Autodesk Fusion 360 part; units mm, degrees
sketch "Sketch1" plane through (0, 0, 0) normal (0, 0, 1) x (1, 0, 0)
  line L0 (0, 0) -> (36, 0)
  line L1 (36, 0) -> (36, 18)
  line L2 (36, 18) -> (0, 18)
  line L3 (0, 18) -> (0, 0)
  dimension "d1" = 36
  dimension "d2" = 18
extrude "Extrude1" add sketch "Sketch1" along normal blind 20
sketch "Sketch2" plane through (0, 0, 20) normal (0, 0, 1) x (-1, 0, 0)
  line L0 (0, -18) -> (0, 0)
  line L1 (0, 0) -> (-36, 0)
  line L2 (-36, 0) -> (-36, -18)
  line L3 (-36, -18) -> (0, -18)
  circle A0 centre (-18, -18) radius 13
  dimension "d5" = 26
extrude "Extrude2" cut sketch "Sketch2" against normal blind 20 contours L3 A0 picked at (-19.0768, -11.2377)
ref_plane "WorkPlane1" through (0, 20, 0) normal (0, 1, 0) x (0, 0, 1)
sketch "Sketch3" plane through (36, 0, 0) normal (1, 0, 0) x (0, 1, 0)
  line L0 (0, 0) -> (18, 0)
  line L1 (18, 0) -> (18, 20)
  line L2 (18, 20) -> (0, 20)
  line L3 (0, 20) -> (0, 0)
  line L4 (18, 20) -> (15, 20)
  line L5 (15, 20) -> (15, 0)
  line L6 (15, 0) -> (18, 0)
  line L7 (18, 0) -> (18, 20)
extrude "Extrude3" add sketch "Sketch3" along normal blind 5 contours L0 L1 L2 L4 L5 L6 L7
sketch "Sketch4" plane through (0, 0, 0) normal (-1, 0, 0) x (0, -1, 0)
  line L0 (-18, 0) -> (0, 0)
  line L1 (0, 0) -> (0, 20)
  line L2 (0, 20) -> (-18, 20)
  line L3 (-18, 20) -> (-18, 0)
  line L4 (-18, 20) -> (-15, 20)
  line L5 (-15, 20) -> (-15, 0)
  line L6 (-15, 0) -> (-18, 0)
  line L7 (-18, 0) -> (-18, 20)
  point P0 (-15, 0)
extrude "Extrude4" add sketch "Sketch4" along normal blind 5 contours L0 L2 L3 L4 L5 L6 L7
sketch "Sketch5" plane through (0, 15, 0) normal (0, -1, 0) x (1, 0, 0)
  line L0 (36, 20) -> (36, 0)
  line L1 (36, 0) -> (41, 0)
  line L2 (41, 0) -> (41, 20)
  line L3 (41, 20) -> (36, 20)
  line L4 (36, 10) -> (46, 10) construction
  circle A0 centre (38.5, 15) radius 1.5
  line L5 (5, 20) -> (5, 0)
  line L6 (18, 10) -> (18, 25) construction
  circle A1 centre (38.5, 5) radius 1.5
  circle A2 centre (-2.5, 15) radius 1.5
  circle A3 centre (-2.5, 5) radius 1.5
  point P0 (0, 20)
  dimension "d13" = 3
  dimension "d14" = 5
  dimension "d15" = 2.5
Check sheet for the modelled part. Datum: model origin and axes. Units: mm. A direction names the side the tool comes from. Round coordinates to 2 decimals unless told otherwise and drop trailing zeros. Write each loop counter-clockwise with the first axis right and the second up, starting at its lowest first coordinate (ties: lowest second). Pieces come first, ordered by that corner, then holes. Notation, with made-up numbers: (69.25, 53) -> (96.25, 53) arc R20 cw to (96.25, 89) -> close; hole circle Ø4 at (-7.5, 44). An arc over 180 degrees is marked (long way). One line per question, with ' | ' between items. Start each with the question number.
1. Set-up check for faces 1 (the face through (36, 7, 10)), 2 (the face through (36, 18, 10)): record each of +Z, -Z, +X, -X, +Y, -Y from which the full face is reachable in a straight line by a thin tool's end or side.
2. Sectioned sample at C-C, the plane x = 18. Record the cut outline in (y, z).
3. Sectioned sample at A-A, the plane y = 5.75. Record the cut outline in (x, z).
4. Sectioned sample at D-D, the plane y = 17. Record the cut outline in (x, z), then the cut area to 3 significant figures.
5. Depth check by flat-ended pin: pin 1 (7.5 mm diameter, centred on y = 7, z = 14.5, fed in from +X); pin 2 (2 mm diameter, centred on x = 9.5, z = 17, fed in from +Y); pin 3 (4 mm diameter, centred on x = 38.5, z = 12, fed in from -Y). Enter the tip coordinate at first touch or a pass-through.
6. Release check for a two-part mould opening along X. For faces 3 (the face through (0, 8, 10)), 4 (the face through (-2, 15, 10)), 5 (the face through (18, 5, 10)) record: +X half, -X half, draft (parallel to the pull), parting line (faces both ways), or undercut.
7. Scan lines: line 1 along X through (y, z) = (3.25, 9.25); line 2 along Y through (x, z) = (37.5, 16.25); line 3 along X through (y, z) = (6.75, 1.5). Record each from-to range of solid material in increasing order. Write a range as from..to.
8. Sectioned sample at B-B, the plane z = 11.75. Record the cut outline in (x, y).
Taken from the geometry:
1) face 1: +Z, -Z, +X, -Y | face 2: +Z, -Z, +X, -X, +Y
2) outline: (0, 0) -> (5, 0) -> (5, 20) -> (0, 20) -> close
3) outline: (0, 0) -> (13.65, 0) -> (13.65, 20) -> (0, 20) -> close; (22.35, 0) -> (36, 0) -> (36, 20) -> (22.35, 20) -> close
4) outline: (-5, 0) -> (5.04, 0) -> (5.04, 20) -> (-5, 20) -> close; (30.96, 0) -> (41, 0) -> (41, 20) -> (30.96, 20) -> close | area: 402 mm^2
5) pin 1: stops at x = 36 | pin 2: stops at y = 9.13 | pin 3: stops at y = 15
6) face 3: -X half | face 4: draft | face 5: undercut
7) line 1: x = 0..36 | line 2: y = 15..18 | line 3: x = 0..11.49, 24.51..36
8) outline: (-5, 15) -> (0, 15) -> (0, 0) -> (36, 0) -> (36, 15) -> (41, 15) -> (41, 18) -> (31, 18) arc R13 cw to (5, 18) -> (-5, 18) -> close
